The listing builds one solid part. Answer for the finished solid, in the listing's coordinates (mm). Face numbers are marked on the shaded views. Give positions to 0.01 mm unless a question says otherwise; leave off trailing zeros. Order: outer loops, then holes, each group sorted by start corner. A loop starts at its lowest first (then second) coordinate and runs counter-clockwise, first axis right, second up. Notation, with made-up numbers: (38.5, 41.25) - (58.5, 41.25) arc R4 cw to (58.5, 46.25) - close; hole circle Ø5 at (10, 81.25). An arc over 180 degrees is marked (long way). Use CSV: the item, a comma, the result in double quotes.
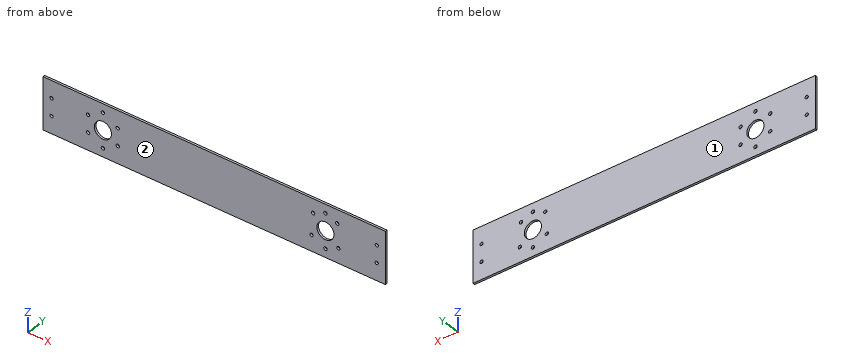
```python
from build123d import *

# Parameters (mm, degrees)
SKETCH1_W               = 508
SKETCH1_H               = 76.2
BOSS_EXTRUDE1_DEPTH     = 3.175
SKETCH3_R               = 2.38125
CUT_EXTRUDE2_DEPTH      = 3.175
SKETCH4_R               = 12.7
CUT_EXTRUDE3_DEPTH      = 1
CUT_EXTRUDE3_DEPTH_BACK = 4.175
SKETCH5_R               = 2.4892
CUT_EXTRUDE4_DEPTH      = 1
CUT_EXTRUDE4_DEPTH_BACK = 4.175


with BuildPart() as part:
    # Sketch1 → Boss-Extrude1 (new body)
    with BuildSketch(Plane(origin=(0, 0, 0), x_dir=(1, 0, 0), z_dir=(0, 1, 0))):
        Rectangle(SKETCH1_W, SKETCH1_H)
    extrude(amount=BOSS_EXTRUDE1_DEPTH)

    # Sketch3 → Cut-Extrude2 (cut)
    with BuildSketch(Plane(origin=(0, 3.175, 0), x_dir=(1, 0, 0), z_dir=(0, 1, 0))):
        with Locations((-241.3, 12.7)):
            Circle(SKETCH3_R)
        with Locations((-241.3, -12.7)):
            Circle(SKETCH3_R)
        with Locations((241.3, -12.7)):
            Circle(SKETCH3_R)
        with Locations((241.3, 12.7)):
            Circle(SKETCH3_R)
    extrude(amount=-CUT_EXTRUDE2_DEPTH, mode=Mode.SUBTRACT)

    # Sketch4 → Cut-Extrude3 (cut, two sides)
    with BuildSketch(Plane(origin=(0, 3.175, 0), x_dir=(1, 0, 0), z_dir=(0, 1, 0))) as cut_extrude3_sk:
        with Locations((-165.1, 0)):
            Circle(SKETCH4_R)
        with Locations((165.1, 0)):
            Circle(SKETCH4_R)
    extrude(amount=CUT_EXTRUDE3_DEPTH, mode=Mode.SUBTRACT)
    extrude(cut_extrude3_sk.sketch, amount=-CUT_EXTRUDE3_DEPTH_BACK, mode=Mode.SUBTRACT)

    # Sketch5 → Cut-Extrude4 (cut, two sides)
    with BuildSketch(Plane(origin=(0, 3.175, 0), x_dir=(1, 0, 0), z_dir=(0, 1, 0))) as cut_extrude4_sk:
        with Locations((165.1, 25.4)):
            Circle(SKETCH5_R)
        with Locations((165.1, -25.4)):
            Circle(SKETCH5_R)
        with Locations((182.702284282, -18.311733617)):
            Circle(SKETCH5_R)
        with Locations((146.781232197, -17.594963659)):
            Circle(SKETCH5_R)
        with Locations((144.478364545, 14.829300427)):
            Circle(SKETCH5_R)
        with Locations((184.428439169, 16.479424725)):
            Circle(SKETCH5_R)
        with Locations((-165.1, 25.4)):
            Circle(SKETCH5_R)
        with Locations((-165.1, -25.4)):
            Circle(SKETCH5_R)
        with Locations((-143.102954744, -12.7)):
            Circle(SKETCH5_R)
        with Locations((-143.102954744, 12.7)):
            Circle(SKETCH5_R)
        with Locations((-187.097045256, 12.7)):
            Circle(SKETCH5_R)
        with Locations((-187.097045256, -12.7)):
            Circle(SKETCH5_R)
    extrude(amount=CUT_EXTRUDE4_DEPTH, mode=Mode.SUBTRACT)
    extrude(cut_extrude4_sk.sketch, amount=-CUT_EXTRUDE4_DEPTH_BACK, mode=Mode.SUBTRACT)


solid = part.part
```
Item 1: Find the intervals of material crossed by line 1 along X through (y, z) = (1.7, -25.4); line 2 along X through (y, z) = (1.35, 1.5); line 3 along Z through (x, y) = (-165.1, 1.4), in increasing order.
Taken from the geometry:
line 1,"-254 to -167.59, -162.61 to 162.61, 167.59 to 254"
line 2,"-254 to -177.71, -152.49 to 152.49, 177.71 to 254"
line 3,"-38.1 to -27.89, -22.91 to -12.7, 12.7 to 22.91, 27.89 to 38.1"
Item 2: The part is cut by section A-A (y = 1). Count the separate pieces of the cut face and the enclosed holes in it, and give its area (3 significant figures).
Taken from the geometry:
separate pieces,"1"
enclosed holes,"18"
area,"37,400 mm^2"
Item 3: The mould has two halves that part along Y. Classify the marked faces 1 and 2: +Y half, -Y half, draft (parallel to the pull), parting line (faces both ways), or undercut.
Taken from the geometry:
face 1,"+Y half"
face 2,"-Y half"
Item 4: The part is cut by section B-B (z = -6). Give the vertices of the cut face in (x, y) (3 decimals).
Taken from the geometry:
outline,"(-254, 0) - (-176.293, 0) - (-176.293, 3.175) - (-254, 3.175) - close; (-153.907, 0) - (153.907, 0) - (153.907, 3.175) - (-153.907, 3.175) - close; (176.293, 0) - (254, 0) - (254, 3.175) - (176.293, 3.175) - close"
